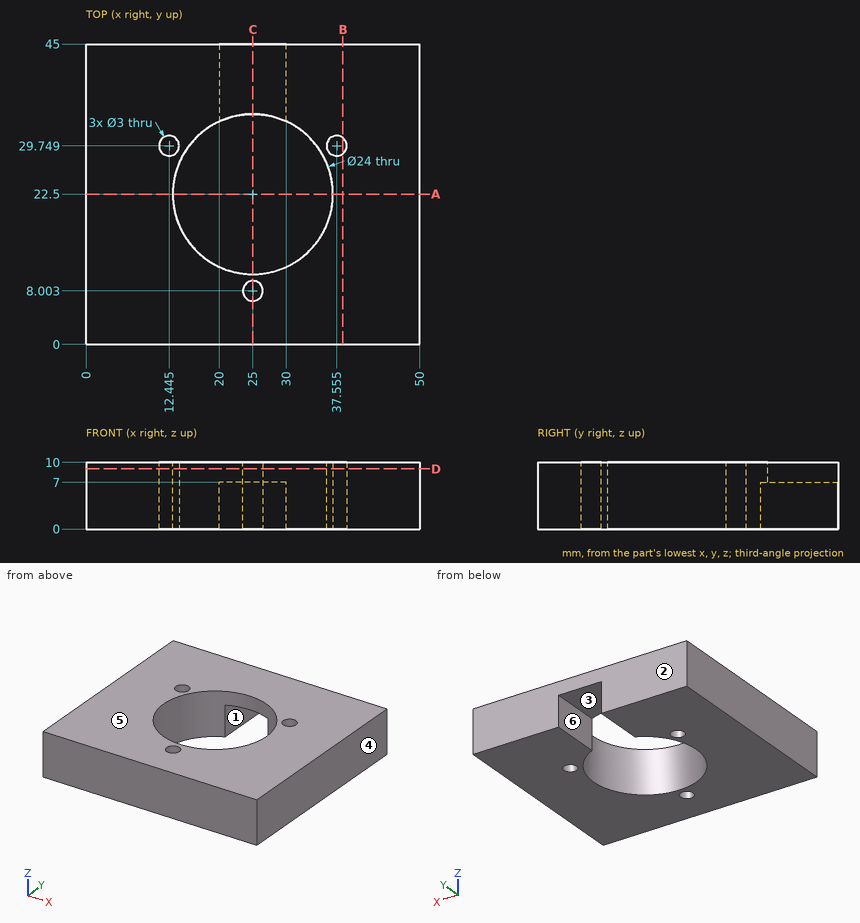
Print and shaded views of the part. All mm, measured from the part's lowest x, y and z. A direction names the side the tool comes from. Coordinates: 2 decimals unless noted, no trailing zeros. Write each loop counter-clockwise with the first axis right and the second up, starting at its lowest first coordinate (ties: lowest second). Pieces come first, ordered by that corner, then holes.
(1) Drill centre lines: probe 1 along X at (y, z) = (22.5, 9); probe 2 along Y at (x, z) = (38, 3.5) (1 decimal); probe 3 along X at (y, z) = (37, 5.5). Where is each one in solid material? Low to high.
(2) Two-plate mould, pull along X, no slides. Class the marked faces 3, 4, 5 and 6: +X half, -X half, draft (parallel to the pull), parting line (faces both ways), or undercut.
(3) Cut at A-A, the plane y = 22.5. List the corners of the cut face in (x, z), and give its area (3 significant figures).
(4) 3-axis set-ups, long thin cutter, end or side, ignore diameter. For the marked faces 1 and 2: which of +Z, -Z, +X, -X, +Y, -Y reach the whole face in a straight line?
(5) Cut at D-D, the plane z = 9. List the corners of the cut face in (x, y) (1 decimal).
(6) Cut at B-B, the plane x = 38.5. List the corners of the cut face in (y, z), and give its area (3 significant figures).
(7) Cut at C-C, the plane x = 25. List the corners of the cut face in (y, z).
Geometry says:
1. probe 1: x = 0 to 13, 37 to 50
1. probe 2: y = 0 to 28.3, 31.2 to 45
1. probe 3: x = 0 to 20, 30 to 50
2. face 3: undercut
2. face 4: +X half
2. face 5: draft
2. face 6: undercut
3. outline: (0, 0) - (13, 0) - (13, 10) - (0, 10) - close; (37, 0) - (50, 0) - (50, 10) - (37, 10) - close
3. area: 260 mm2
4. face 1: -Z, +Y
4. face 2: +Z, -Z, +X, -X, +Y
5. outline: (0, 0) - (50, 0) - (50, 45) - (0, 45) - close; hole circle Ø3 at (12.4, 29.7); hole circle Ø24 at (25, 22.5); hole circle Ø3 at (25, 8); hole circle Ø3 at (37.6, 29.7)
6. outline: (0, 0) - (28.58, 0) - (28.58, 10) - (0, 10) - close; (30.91, 0) - (45, 0) - (45, 10) - (30.91, 10) - close
6. area: 427 mm2
7. outline: (0, 0) - (6.5, 0) - (6.5, 10) - (0, 10) - close; (9.5, 0) - (10.5, 0) - (10.5, 10) - (9.5, 10) - close; (34.5, 7) - (45, 7) - (45, 10) - (34.5, 10) - close
